Part model, mm, in its own coordinate system. A direction names the side the tool comes from. Round coordinates to 2 decimals unless told otherwise and drop trailing zeros. Order: outer loops, then holes, each group sorted by start corner. A loop starts at its lowest first (then second) coordinate and runs counter-clockwise, first axis right, second up. Notation, with made-up numbers: (65, 77) - (72, 77) arc R21 cw to (72, 116) - close; hole circle Ø11 at (57, 25). An arc over 180 degrees is marked (long way). Return JSON: item names as keys, results as strings. Group by question number.
Item 1: Saw through at C-C on y = 44.4. List the corners of the cut face in (x, z) (3 decimals).
Item 2: Saw through at B-B on z = 1.25. State how many separate pieces and enclosed holes the cut face has, and give its area (3 significant figures).
Item 3: Saw through at A-A on y = 0. List the corners of the cut face in (x, z) (3 decimals).
Item 4: Tool access for faces 5 (the face through (-10, 2.159, 6)), 6 (the face through (0.32, 41.963, 4.829)): list every direction of +Z, -Z, +X, -X, +Y, -Y with a clear straight run to the whole face (end or side of a thin tool).
Item 5: Drop flat-ended pins along their axis: pin 1 (5 mm diameter, centred on x = 9.5, z = -3.5, fed in from -Y); pin 2 (0.6 mm diameter, centred on y = 5.5, z = 8, fed in from -X); pin 3 (1.5 mm diameter, centred on y = -6, z = 8, fed in from +X); pin 4 (6.5 mm diameter, centred on x = -12.7, y = 44.4, fed in from +Z) (3 decimals). Give the stop position or say it passes through.
Item 6: Two-plate mould, pull along Y, no slides. Class faces 1 (the face through (0, -19, 5)), 2 (the face through (0, 35, 0)), 3 (the face through (0, -14, 9)), 4 (the face through (-14.986, 0, 9)): released by +Y, released by -Y, zero draft, split by the parting line, or undercut.
Item 7: Probe probe 1 along Y at (x, z) = (0, 6.75); probe 2 along X at (y, z) = (57.1, 6.5); probe 3 along Y at (x, z) = (14, 3). List the from-to ranges inside material, lowest first.
```python
from build123d import *

# Parameters (mm, degrees)
SKETCH1_W                    = 38
SKETCH1_H                    = 38
BOSS_EXTRUDE1_DEPTH          = 9.525
F_36_0_1065_DIAMETER_HOLE2_D = 2.7051
SKETCH8_W                    = 38.1
SKETCH8_H                    = 9.525
BOSS_EXTRUDE2_DEPTH          = 50.8
F_10_0_1935_DIAMETER_HOLE1_D = 4.9149
CUT_EXTRUDE2_DEPTH           = 1.905
CUT_EXTRUDE4_START           = 1.905
SKETCH13_W                   = 14.732
SKETCH13_H                   = 14.732
CUT_EXTRUDE4_DEPTH           = 4.7498
SKETCH14_W                   = 23.5204
SKETCH14_H                   = 4.318
CUT_EXTRUDE5_DEPTH           = 2.8448
SKETCH15_R                   = 12.7
BOSS_EXTRUDE3_DEPTH          = 6.9596
SKETCH12_R                   = 7.239
CUT_EXTRUDE3_DEPTH           = 74.807230243
CHAMFER1_SIZE2               = 3.245314778
CHAMFER1_SIZE                = 6.9596
FILLET4_R                    = 2.54
LPATTERN1_COUNT              = 3
LPATTERN1_PITCH              = 12.7


with BuildPart() as part:
    # Sketch1 → Boss-Extrude1 (new body)
    with BuildSketch(Plane(origin=(0, 0, 0), x_dir=(0, 1, 0), z_dir=(0, 0, 1))):
        Rectangle(SKETCH1_W, SKETCH1_H)
    extrude(amount=BOSS_EXTRUDE1_DEPTH)

    # #36 (0.1065) Diameter Hole2 (through all)
    with Locations(Plane.XY.offset(9.525)):
        with Locations((-14, -14), (14, -14), (14, 14), (-14, 14)):
            Hole(F_36_0_1065_DIAMETER_HOLE2_D / 2)

    # Sketch8 → Boss-Extrude2 (add)
    with BuildSketch(Plane(origin=(0, 19, 0), x_dir=(-1, 0, 0), z_dir=(0, 1, 0))):
        with Locations((0, 4.7625)):
            Rectangle(SKETCH8_W, SKETCH8_H)
    extrude(amount=BOSS_EXTRUDE2_DEPTH)

    # #10 (0.1935) Diameter Hole1 (through all)
    with Locations(Plane(origin=(0, 0, 0), x_dir=(1, 0, 0), z_dir=(0, 0, -1))):
        with Locations((-12.7, -57.1), (0, -57.1), (12.7, -57.1), (25.4, -57.1), (38.1, -57.1)):
            f_10_0_1935_diameter_hole1 = Hole(F_10_0_1935_DIAMETER_HOLE1_D / 2)

    # Sketch11 → Cut-Extrude2 (cut)
    with BuildSketch(Plane.XY.offset(9.525)):
        with BuildLine():
            Line((11.69495, -14), (-11.69495, -14))
            ThreePointArc((-11.69495, -14), (-12.76702064, -12.052432953), (-14.986, -11.916479061))
            Line((-14.986, -11.916479061), (-14.986, 11.916479061))
            ThreePointArc((-14.986, 11.916479061), (-12.76702064, 12.052432953), (-11.69495, 14))
            Line((-11.69495, 14), (11.69495, 14))
            ThreePointArc((11.69495, 14), (12.76702064, 12.052432953), (14.986, 11.916479061))
            Line((14.986, 11.916479061), (14.986, -11.916479061))
            ThreePointArc((14.986, -11.916479061), (12.76702064, -12.052432953), (11.69495, -14))
        make_face()
    extrude(amount=-CUT_EXTRUDE2_DEPTH, mode=Mode.SUBTRACT)

    # Sketch13 → Cut-Extrude4 (cut)
    with BuildSketch(Plane.XY.offset(7.62).offset(CUT_EXTRUDE4_START)):
        Rectangle(SKETCH13_W, SKETCH13_H)
    extrude(amount=-CUT_EXTRUDE4_DEPTH, mode=Mode.SUBTRACT)

    # Sketch14 → Cut-Extrude5 (cut)
    with BuildSketch(Plane.XY.offset(7.62)):
        Rectangle(SKETCH14_W, SKETCH14_H)
    extrude(amount=-CUT_EXTRUDE5_DEPTH, mode=Mode.SUBTRACT)

    # Sketch15 → Boss-Extrude3 (add)
    with BuildSketch(Plane(origin=(0, 0, 0), x_dir=(1, 0, 0), z_dir=(0, 0, -1))):
        with Locations(Location((0, 0, 0), (0, 0, 180))):
            Circle(SKETCH15_R)
    extrude(amount=BOSS_EXTRUDE3_DEPTH)

    # Sketch12 → Cut-Extrude3 (cut, through all)
    with BuildSketch(Plane.XY.offset(7.62)):
        Circle(SKETCH12_R)
    extrude(amount=-CUT_EXTRUDE3_DEPTH, mode=Mode.SUBTRACT)

    # Chamfer1
    chamfer1_edges = [part.edges().sort_by_distance(p)[0] for p in [
        (12.7, 0, -6.9596),
    ]]
    chamfer1_side = [part.faces().sort_by_distance(p)[0] for p in [
        (12.7, 0, -6.894693704),
    ]]
    chamfer(chamfer1_edges, length=CHAMFER1_SIZE - 0.0001, length2=CHAMFER1_SIZE2 - 0.0001, reference=chamfer1_side[0])  # a hair under: the kernel refuses the full size

    # Fillet3: read off the stored shape, not the designer's step
    # Fillet3 outline → Fillet3 (revolve)
    with BuildSketch(Plane.XZ):
        with BuildLine():
            Line((11.161307538, 0), (11.161307538, -3.299736634))
            ThreePointArc((11.161307538, -3.299736634), (13.270189279, -0.895017887), (16.340856541, 0))
            Line((16.340856541, 0), (11.161307538, 0))
        make_face()
    revolve(axis=Axis((0, 0, 0), (0, 0, 1)))

    # Fillet4
    fillet4_edges = [part.edges().sort_by_distance(p)[0] for p in [
        (9.454785222, 0, -6.9596),
    ]]
    fillet(fillet4_edges, radius=FILLET4_R)

    # LPattern1: #10 (0.1935) Diameter Hole1 ×3
    with Locations(*[(0, -i * LPATTERN1_PITCH, 0) for i in range(1, LPATTERN1_COUNT)]):
        add(f_10_0_1935_diameter_hole1, mode=Mode.SUBTRACT)


solid = part.part
```
Filled in:
{
 "1": {"outline": "(-19.05, 0) - (-15.157, 0) - (-15.157, 9.525) - (-19.05, 9.525) - close; (-10.243, 0) - (-2.457, 0) - (-2.457, 9.525) - (-10.243, 9.525) - close; (2.457, 0) - (10.243, 0) - (10.243, 9.525) - (2.457, 9.525) - close; (15.157, 0) - (19.05, 0) - (19.05, 9.525) - (15.157, 9.525) - close"},
 "2": {"separate pieces": "1", "enclosed holes": "14", "area": "3,020 mm^2"},
 "3": {"outline": "(-19, 0) - (-16.341, 0) arc R5.715 cw to (-11.173, -3.275) - (-10.139, -5.493) arc R2.54 ccw to (-7.837, -6.96) - (-7.239, -6.96) - (-7.239, 4.775) - (-11.76, 4.775) - (-11.76, 7.62) - (-14.986, 7.62) - (-14.986, 9.525) - (-19, 9.525) - close; (7.239, -6.96) - (7.837, -6.96) arc R2.54 ccw to (10.139, -5.493) - (11.173, -3.275) arc R5.715 cw to (16.341, 0) - (19, 0) - (19, 9.525) - (14.986, 9.525) - (14.986, 7.62) - (11.76, 7.62) - (11.76, 4.775) - (7.239, 4.775) - close"},
 "4": {"face 5": "+Z", "face 6": "+Z, -Z"},
 "5": {"pin 1": "stops at y = -9.62", "pin 2": "stops at x = -19", "pin 3": "stops at x = 19", "pin 4": "stops at z = 9.525"},
 "6": {"face 1": "released by -Y", "face 2": "zero draft", "face 3": "undercut", "face 4": "undercut"},
 "7": {"probe 1": "y = -19 to -7.37, 7.37 to 29.24, 34.16 to 41.94, 46.86 to 54.64, 59.56 to 69.8", "probe 2": "x = -19.05 to -15.16, -10.24 to -2.46, 2.46 to 10.24, 15.16 to 19.05", "probe 3": "y = -19 to -15.35, -12.65 to 12.65, 15.35 to 29.61, 33.79 to 42.31, 46.49 to 55.01, 59.19 to 69.8"}
}
